Verification items for this drawing (mm, ordinates from the low corner). A direction names the side the tool comes from. Coordinates: 2 decimals unless noted, no trailing zeros. Loops run counter-clockwise (first coordinate to the right, second up) from the corner with the lowest first, then second, coordinate; pieces in that order, holes last. Notation, with made-up numbers: M 80,-29 L 109,-29 A8 ccw 109,-17 Z; hole C 1.25,53 d8. An arc over 180 degrees is marked long. Use CSV: the item, a comma, the result in double quotes.
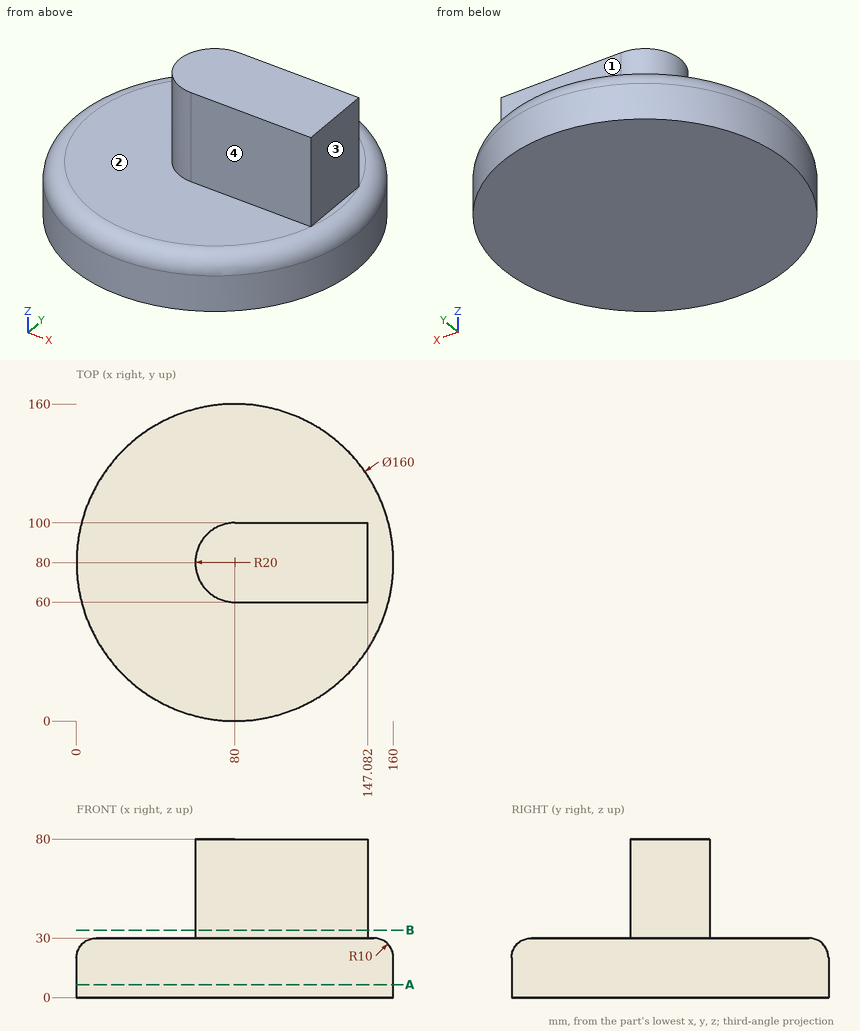
1. Thickness scan on line 1 (Z direction, x = 131, y = 116); line 2 (Y direction, x = 146, z = 49); line 3 (X direction, y = 78, z = 12) (3 decimals). Record the ranges inside material, lowest first. Write a range as [from, to].
The answers:
line 1,"[0, 30]"
line 2,"[60, 100]"
line 3,"[0.025, 159.975]"
2. Gauge pin test, flat ends, axial feed: P1, Ø1.5, axis at y = 126.5, z = 27.5, coming from the +X side; P2, Ø0.9, axis at x = 148.5, y = 85.5, coming from the +Z side; P3, Ø25, axis at x = 110.5, z = 52, coming from the +Y side. Record the tip position at first contact, or that the pin passes through.
The answers:
P1,"x = 142.01"
P2,"z = 30"
P3,"y = 100"
3. Section check A-A, the plane z = 6.5. Record the cut outline in (x, y).
The answers:
outline,"C 80,80 d160"
4. Section check B-B, the plane z = 34. Record the cut outline in (x, y), plus the area to 3 significant figures.
The answers:
outline,"M 80,60 L 147.08,60 L 147.08,100 L 80,100 A20 ccw Z"
area,"3,310 mm^2"
5. Set-up check for the marked faces 1, 2, 3 and 4: record each of +Z, -Z, +X, -X, +Y, -Y from which the full face is reachable in a straight line by a thin tool's end or side.
The answers:
face 1,"+Z, +X, -X, +Y"
face 2,"+Z, -X"
face 3,"+Z, +X, +Y, -Y"
face 4,"+Z, +X, -X, -Y"
